Autodesk Inventor part; units mm, degrees
ref_plane "Work Plane2" through (0, 0, 10) normal (0, 0, 1) x (1, 0, 0)
ref_plane "Work Plane8" through (0, 0, 0) normal (0.9510565, 0.309017, 0) x (0, 0, 1)
ref_plane "Work Plane9" through (0, 0, 0) normal (1, 0, 0) x (0, 1, 0)
sketch "Sketch1" plane through (0, 0, 0) normal (0, 0, 1) x (1, 0, 0)
  circle A0 centre (0, 0) radius 3.0354
  dimension "d0" = 6.0708
extrude "Extrusion1" add sketch "Sketch1" along normal blind 20
ref_plane "Work Plane2" through (0, 0, 10) normal (0, 0, 1) x (1, 0, 0)
sketch "Sketch2" plane through (0, 0, 0) normal (0, 0, -1) x (-1, 0, 0)
  circle A0 centre (0, 0) radius 3.0354
  circle A1 centre (0, 0) radius 2.5295
  dimension "d3" = 5.059
surface extrude "Pitch Diameter" sketch "Sketch2" against normal through all shown no curves A1
ref_plane "Work Plane8" through (0, 0, 0) normal (0.9510565, 0.309017, 0) x (0, 0, 1)
ref_plane "Work Plane9" through (0, 0, 0) normal (1, 0, 0) x (0, 1, 0)
spur gear teeth "Spur Gear" teeth 10 pitch diameter 5.059 tip diameter 6.0708 root diameter 3.7942 face width 20 start plane through (0, 0, 0) normal (0, 0, -1) x (-1, 0, 0)
sketch "Sketch3" plane through (0, 0, 20) normal (0, 0, 1) x (1, 0, 0)
  arc A0 (-1.9713, 2.3081) -> (-1.4426, 1.2321) centre (0.7208, 2.9631) ccw
  arc A1 (-1.4426, 1.2321) -> (-1.6176, 0.9912) centre (0, 0) ccw
  arc A2 (-1.6176, 0.9912) -> (-2.8043, 1.1616) centre (-2.5953, -1.6011) ccw
  arc A3 (-2.8043, 1.1616) -> (-2.9515, 0.7086) centre (0, 0) ccw
  arc A4 (-2.9515, 0.7086) -> (-1.8913, 0.1488) centre (-1.1585, 2.8208) ccw
  arc A5 (-1.8913, 0.1488) -> (-1.8913, -0.1488) centre (0, 0) ccw
  arc A6 (-1.8913, -0.1488) -> (-2.9515, -0.7086) centre (-1.1585, -2.8208) ccw
  arc A7 (-2.9515, -0.7086) -> (-2.8043, -1.1616) centre (0, 0) ccw
  arc A8 (-2.8043, -1.1616) -> (-1.6176, -0.9912) centre (-2.5953, 1.6011) ccw
  arc A9 (-1.6176, -0.9912) -> (-1.4426, -1.2321) centre (0, 0) ccw
  arc A10 (-1.4426, -1.2321) -> (-1.9713, -2.3081) centre (0.7208, -2.9631) ccw
  arc A11 (-1.9713, -2.3081) -> (-1.586, -2.5881) centre (0, 0) ccw
  arc A12 (-1.586, -2.5881) -> (-0.726, -1.7527) centre (-3.0408, -0.2301) ccw
  arc A13 (-0.726, -1.7527) -> (-0.4429, -1.8447) centre (0, 0) ccw
  arc A14 (-0.4429, -1.8447) -> (-0.2382, -3.026) centre (2.3248, -1.9735) ccw
  arc A15 (-0.2382, -3.026) -> (0.2382, -3.026) centre (0, 0) ccw
  arc A16 (0.2382, -3.026) -> (0.4429, -1.8447) centre (-2.3248, -1.9735) ccw
  arc A17 (0.4429, -1.8447) -> (0.726, -1.7527) centre (0, 0) ccw
  arc A18 (0.726, -1.7527) -> (1.586, -2.5881) centre (3.0408, -0.2301) ccw
  arc A19 (1.586, -2.5881) -> (1.9713, -2.3081) centre (0, 0) ccw
  arc A20 (1.9713, -2.3081) -> (1.4426, -1.2321) centre (-0.7208, -2.9631) ccw
  arc A21 (1.4426, -1.2321) -> (1.6176, -0.9912) centre (0, 0) ccw
  arc A22 (1.6176, -0.9912) -> (2.8043, -1.1616) centre (2.5953, 1.6011) ccw
  arc A23 (2.8043, -1.1616) -> (2.9515, -0.7086) centre (0, 0) ccw
  arc A24 (2.9515, -0.7086) -> (1.8913, -0.1488) centre (1.1585, -2.8208) ccw
  arc A25 (1.8913, -0.1488) -> (1.8913, 0.1488) centre (0, 0) ccw
  arc A26 (1.8913, 0.1488) -> (2.9515, 0.7086) centre (1.1585, 2.8208) ccw
  arc A27 (2.9515, 0.7086) -> (2.8043, 1.1616) centre (0, 0) ccw
  arc A28 (2.8043, 1.1616) -> (1.6176, 0.9912) centre (2.5953, -1.6011) ccw
  arc A29 (1.6176, 0.9912) -> (1.4426, 1.2321) centre (0, 0) ccw
  arc A30 (1.4426, 1.2321) -> (1.9713, 2.3081) centre (-0.7208, 2.9631) ccw
  arc A31 (1.9713, 2.3081) -> (1.586, 2.5881) centre (0, 0) ccw
  arc A32 (1.586, 2.5881) -> (0.726, 1.7527) centre (3.0408, 0.2301) ccw
  arc A33 (0.726, 1.7527) -> (0.4429, 1.8447) centre (0, 0) ccw
  arc A34 (0.4429, 1.8447) -> (0.2382, 3.026) centre (-2.3248, 1.9735) ccw
  arc A35 (0.2382, 3.026) -> (-0.2382, 3.026) centre (0, 0) ccw
  arc A36 (-0.2382, 3.026) -> (-0.4429, 1.8447) centre (2.3248, 1.9735) ccw
  arc A37 (-0.4429, 1.8447) -> (-0.726, 1.7527) centre (0, 0) ccw
  arc A38 (-0.726, 1.7527) -> (-1.586, 2.5881) centre (-3.0408, 0.2301) ccw
  arc A39 (-1.586, 2.5881) -> (-1.9713, 2.3081) centre (0, 0) ccw
  circle A40 centre (0, 0) radius 1
  dimension "d49" = 2
ref_plane "Work Plane11" through (-4.7906, 1.2372, 4) normal (0, 0, 1) x (0.9749279, -0.2225209, 0)
extrude "Extrusion2" cut sketch "Sketch3" against normal up to surface (16 mm away) contours A39 A38 A37 A36 A35 A34 A33 A32 A31 A30 A29 A28 A27 A26 A25 A24 A23 A22 A21 A20 A19 A18 A17 A16 A15 A14 A13 A12 A11 A10 A9 A8 A7 A6 A5 A4 A3 A2 A1 A0 | A40
extrude "Extrusion3" cut sketch "Sketch3" against normal through all contours A40
sketch "Sketch4" plane through (0, 0, 4) normal (0, 0, 1) x (1, 0, 0)
  circle A0 centre (0, 0) radius 1
  arc A1 (-1.6176, 0.9912) -> (-2.8043, 1.1616) centre (-2.5953, -1.6011) ccw
  arc A2 (-2.8043, 1.1616) -> (-2.9515, 0.7086) centre (0, 0) ccw
  arc A3 (-2.9515, 0.7086) -> (-1.8913, 0.1488) centre (-1.1585, 2.8208) ccw
  arc A4 (-1.8913, 0.1488) -> (-1.8913, -0.1488) centre (0, 0) ccw
  arc A5 (-1.8913, -0.1488) -> (-2.9515, -0.7086) centre (-1.1585, -2.8208) ccw
  arc A6 (-2.9515, -0.7086) -> (-2.8043, -1.1616) centre (0, 0) ccw
  arc A7 (-2.8043, -1.1616) -> (-1.6176, -0.9912) centre (-2.5953, 1.6011) ccw
  arc A8 (-1.6176, -0.9912) -> (-1.4426, -1.2321) centre (0, 0) ccw
  arc A9 (-1.4426, -1.2321) -> (-1.9713, -2.3081) centre (0.7208, -2.9631) ccw
  arc A10 (-1.9713, -2.3081) -> (-1.586, -2.5881) centre (0, 0) ccw
  arc A11 (-1.586, -2.5881) -> (-0.726, -1.7527) centre (-3.0408, -0.2301) ccw
  arc A12 (-0.726, -1.7527) -> (-0.4429, -1.8447) centre (0, 0) ccw
  arc A13 (-0.4429, -1.8447) -> (-0.2382, -3.026) centre (2.3248, -1.9735) ccw
  arc A14 (-0.2382, -3.026) -> (0.2382, -3.026) centre (0, 0) ccw
  arc A15 (0.2382, -3.026) -> (0.4429, -1.8447) centre (-2.3248, -1.9735) ccw
  arc A16 (0.4429, -1.8447) -> (0.726, -1.7527) centre (0, 0) ccw
  arc A17 (0.726, -1.7527) -> (1.586, -2.5881) centre (3.0408, -0.2301) ccw
  arc A18 (1.586, -2.5881) -> (1.9713, -2.3081) centre (0, 0) ccw
  arc A19 (1.9713, -2.3081) -> (1.4426, -1.2321) centre (-0.7208, -2.9631) ccw
  arc A20 (1.4426, -1.2321) -> (1.6176, -0.9912) centre (0, 0) ccw
  arc A21 (1.6176, -0.9912) -> (2.8043, -1.1616) centre (2.5953, 1.6011) ccw
  arc A22 (2.8043, -1.1616) -> (2.9515, -0.7086) centre (0, 0) ccw
  arc A23 (2.9515, -0.7086) -> (1.8913, -0.1488) centre (1.1585, -2.8208) ccw
  arc A24 (1.8913, -0.1488) -> (1.8913, 0.1488) centre (0, 0) ccw
  arc A25 (1.8913, 0.1488) -> (2.9515, 0.7086) centre (1.1585, 2.8208) ccw
  arc A26 (2.9515, 0.7086) -> (2.8043, 1.1616) centre (0, 0) ccw
  arc A27 (2.8043, 1.1616) -> (1.6176, 0.9912) centre (2.5953, -1.6011) ccw
  arc A28 (1.6176, 0.9912) -> (1.4426, 1.2321) centre (0, 0) ccw
  arc A29 (1.4426, 1.2321) -> (1.9713, 2.3081) centre (-0.7208, 2.9631) ccw
  arc A30 (1.9713, 2.3081) -> (1.586, 2.5881) centre (0, 0) ccw
  arc A31 (1.586, 2.5881) -> (0.726, 1.7527) centre (3.0408, 0.2301) ccw
  arc A32 (0.726, 1.7527) -> (0.4429, 1.8447) centre (0, 0) ccw
  arc A33 (0.4429, 1.8447) -> (0.2382, 3.026) centre (-2.3248, 1.9735) ccw
  arc A34 (0.2382, 3.026) -> (-0.2382, 3.026) centre (0, 0) ccw
  arc A35 (-0.2382, 3.026) -> (-0.4429, 1.8447) centre (2.3248, 1.9735) ccw
  arc A36 (-0.4429, 1.8447) -> (-0.726, 1.7527) centre (0, 0) ccw
  arc A37 (-0.726, 1.7527) -> (-1.586, 2.5881) centre (-3.0408, 0.2301) ccw
  arc A38 (-1.586, 2.5881) -> (-1.9713, 2.3081) centre (0, 0) ccw
  arc A39 (-1.9713, 2.3081) -> (-1.4426, 1.2321) centre (0.7208, 2.9631) ccw
  arc A40 (-1.4426, 1.2321) -> (-1.6176, 0.9912) centre (0, 0) ccw
extrude "Extrusion4" cut sketch "Sketch4" against normal blind 1
equation "\"d0\" = da_da"
equation "\"d1\" = da_b"
equation "\"d3\" = da_d"
equation "\"d16\" = da_aw"
equation "\"d43\" = da_aw"
equation "\"d46\" = da_aw"
properties part number "Spur Gear1" material "Steel"
Input: part model. Units: mm. Frame: model coordinates. A direction names the side the tool comes from. Coordinates: 2 decimals unless noted, no trailing zeros. Loops run counter-clockwise (first coordinate to the right, second up) from the corner with the lowest first, then second, coordinate; pieces in that order, holes last.
Q1. Contact query for a flat-ended pin moving along its axis: pin 1 (1.6 mm diameter, centred on x = 0, y = 0, fed in from -Z). Output: stop coordinate, or through.
Q2. Cut plane B-B (y = -0.25). Output: boundary loops of the cut face in (x, z).
Q3. Set-up query: faces 1 (the face through (1.1, 2.21, 1.48)), 2 (the face through (2.46, 0.375, 1.479)), 3 (the face through (2.21, -1.143, 1.479)), 4 (the face through (-1.77, -1.75, 1.48)). Return all of +Z, -Z, +X, -X, +Y, -Y with unobstructed straight access to the full face (end or side cutting, diameter ignored); none if empty.
Q4. Cut plane A-A (x = 0). Output: boundary loops of the cut face in (y, z), then the cut area to 3 significant figures.
Q5. Draft query along Y for faces 5 (the face through (-2.21, 1.143, 1.479)), 6 (the face through (-1.116, 2.223, 1.479)), 7 (the face through (-1, 1, 3)), 8 (the face through (2.445, -0.367, 1.479)). Return one class per face: +Y half, -Y half, draft (parallel to the pull), parting line (faces both ways), or undercut.
Q6. Material intervals for line 1 (Y direction, x = 0, z = 1); line 2 (X direction, y = 2.25, z = 0.55); line 3 (X direction, y = 0.5, z = 1), sorted ascending.
Working result:
1. pin 1: passes through
2. outline: (-2.19, 0) - (-0.97, 0) - (-0.97, 3) - (-2.19, 3) - close; (0.97, 0) - (2.19, 0) - (2.19, 3) - (0.97, 3) - close
3. face 1: +Z, -Z, +Y
3. face 2: +Z, -Z, +X
3. face 3: +Z, -Z
3. face 4: +Z, -Z, -X
4. outline: (-3.04, 0) - (-1, 0) - (-1, 3) - (-3.04, 3) - close; (1, 0) - (3.04, 0) - (3.04, 3) - (1, 3) - close
4. area: 12.2 mm2
5. face 5: undercut
5. face 6: +Y half
5. face 7: draft
5. face 8: undercut
6. line 1: y = -3.04 to -1, 1 to 3.04
6. line 2: x = -1.96 to -1.14, -0.43 to 0.43, 1.14 to 1.96
6. line 3: x = -2.67 to -0.87, 0.87 to 2.67
